```python
from build123d import *


with BuildPart() as f1:
    # F0 (on Right) → F1 (revolve)
    with BuildSketch(Plane.YZ):
        Polygon((-18.7706, 15.1765), (0, 15.1765), (18.7706, 15.1765), (18.7706, 20.9804), (31.4706, 20.9804), (31.4706, 49.3522), (13.1445, 49.3522), (13.1445, 44.8818), (-13.1445, 44.8818), (-13.1445, 49.3522), (-31.4706, 49.3522), (-31.4706, 20.9804), (-18.7706, 20.9804), align=None)
    revolve(axis=Axis((0, -0.984378, 0), (0, 1, 0)))


solid = f1.part
```
Here's how the part is built. I have some questions about the finished solid (model axes, mm). A direction names the side the tool comes from. Coordinates: 2 decimals unless noted, no trailing zeros. Order: outer loops, then holes, each group sorted by start corner. A loop starts at its lowest first (then second) coordinate and runs counter-clockwise, first axis right, second up. Notation, with made-up numbers: (87.5, 49.5) - (126.5, 49.5) arc R18 cw to (126.5, 66.5) - close; hole circle Ø11 at (58.5, -24.5). An arc over 180 degrees is marked (long way). One line per question, with ' | ' between items. Start each with the question number.
1. If we section it at A-A (x = 0): Write out the boundary of the cut face in (y, z).
2. If we section it at C-C (y = -11.5): Write out the boundary of the cut face in (x, z).
3. I'm going to push flat-ended pins straight in: pin 1 Ø6 at (x, y) = (35.5, 4) entering from +Z; pin 2 Ø4 at (y, z) = (4.5, -36.5) entering from +X; pin 3 Ø4 at (y, z) = (7, 6) entering from +X. Where does each tip first touch, or does it pass through?
4. If we section it at B-B (z = 0): Write out the boundary of the cut face in (x, y), and give its area (3 significant figures).
5. If we mould it in two halves opening along Z, with no side actions, what happens to faces 1 (the flat face through (-21.2, -31.471, -0.7)), 2 (the cylindrical face through (4.559, 0.263, 14.476)), 3 (the flat face through (11, 18.771, -11)), 4 (the cylindrical face through (-30.03, -22.436, -39.164))? For each: released by +Z, released by -Z, zero draft, split by the parting line, or undercut.
6. Which directions (+Z, -Z, +X, -X, +Y, -Y) give clear straight access to the entire face, cutting with the end or side of a thin tool? Please do faces 5 (the flat face through (-21.2, 31.471, 0.7)), 6 (the cylindrical face through (0.92, 25.21, -20.96)), 7 (the cylindrical face through (0.92, -25.03, -20.96)), 8 (the cylindrical face through (-30.03, 22.179, -39.164)), 9 (the flat face through (-44, 13.144, 11)).
7. If we section it at D-D (z = -26): Write out the boundary of the cut face in (x, y).
8. Please list where these lines run through material, in increasing order: line 1 along X through (y, z) = (-25, 0); line 2 along X through (y, z) = (11.5, 11); line 3 along Y through (x, z) = (0.5, 17). Write a range as [from, to].
Model answer:
1) outline: (-31.47, -49.35) - (-13.14, -49.35) - (-13.14, -44.88) - (13.14, -44.88) - (13.14, -49.35) - (31.47, -49.35) - (31.47, -20.98) - (18.77, -20.98) - (18.77, -15.18) - (-18.77, -15.18) - (-18.77, -20.98) - (-31.47, -20.98) - close; (-31.47, 20.98) - (-18.77, 20.98) - (-18.77, 15.18) - (18.77, 15.18) - (18.77, 20.98) - (31.47, 20.98) - (31.47, 49.35) - (13.14, 49.35) - (13.14, 44.88) - (-13.14, 44.88) - (-13.14, 49.35) - (-31.47, 49.35) - close
2) outline: circle Ø89.76 at (0, 0); hole circle Ø30.35 at (0, 0)
3) pin 1: stops at z = 30.95 | pin 2: stops at x = 28.71 | pin 3: stops at x = 44.7
4) outline: (-49.35, -31.47) - (-20.98, -31.47) - (-20.98, -18.77) - (-15.18, -18.77) - (-15.18, 18.77) - (-20.98, 18.77) - (-20.98, 31.47) - (-49.35, 31.47) - (-49.35, 13.14) - (-44.88, 13.14) - (-44.88, -13.14) - (-49.35, -13.14) - close; (15.18, -18.77) - (20.98, -18.77) - (20.98, -31.47) - (49.35, -31.47) - (49.35, -13.14) - (44.88, -13.14) - (44.88, 13.14) - (49.35, 13.14) - (49.35, 31.47) - (20.98, 31.47) - (20.98, 18.77) - (15.18, 18.77) - close | area: 3,770 mm²
5) face 1: zero draft | face 2: undercut | face 3: undercut | face 4: split by the parting line
6) face 5: +Z, -Z, +X, -X, +Y | face 6: +Y | face 7: -Y | face 8: +Y, -Y | face 9: none
7) outline: (-41.95, -31.47) - (41.95, -31.47) - (41.95, -13.14) - (36.58, -13.14) - (36.58, 13.14) - (41.95, 13.14) - (41.95, 31.47) - (-41.95, 31.47) - (-41.95, 13.14) - (-36.58, 13.14) - (-36.58, -13.14) - (-41.95, -13.14) - close
8) line 1: x = [-49.35, -20.98], [20.98, 49.35] | line 2: x = [-43.51, -10.46], [10.46, 43.51] | line 3: y = [-18.77, 18.77]
